Geometry check sheet. Reference: the model listing, model coordinates, mm. Face numbers are marked on the shaded views. A direction names the side the tool comes from. Round coordinates to 2 decimals unless told otherwise and drop trailing zeros. Loops run counter-clockwise (first coordinate to the right, second up) from the corner with the lowest first, then second, coordinate; pieces in that order, holes last. Notation, with made-up numbers: (-2.75, 50.25) -> (18.25, 50.25) arc R20 cw to (18.25, 86.25) -> close; hole circle Ø2 at (30, 10.25). An arc over 180 degrees is marked (long way). Use one line per item in the form item = value.
from build123d import *

# Parameters (mm, degrees)
BOSS_EXTRUDE1_DEPTH = 50
SKETCH2_W           = 25
SKETCH2_H           = 10
CUT_EXTRUDE1_DEPTH  = 84.815273071


with BuildPart() as part:
    # Sketch1 → Boss-Extrude1 (new body)
    with BuildSketch(Plane(origin=(0, 0, 0), x_dir=(0, 0, -1), z_dir=(1, 0, 0))):
        Polygon((0, 0), (30, 0), (30, 10), (20, 10), (20, 20), (50, 20), (50, 10), (40, 10), (40, 0), (70, 0), (70, 30), (45, 30), (45, 50), (25, 50), (25, 30), (0, 30), align=None)
    extrude(amount=-BOSS_EXTRUDE1_DEPTH)

    # Sketch2 → Cut-Extrude1 (cut, through all)
    with BuildSketch(Plane.XY.offset(-25)):
        with Locations((-25, 45)):
            Rectangle(SKETCH2_W, SKETCH2_H)
    extrude(amount=-CUT_EXTRUDE1_DEPTH, mode=Mode.SUBTRACT)


solid = part.part
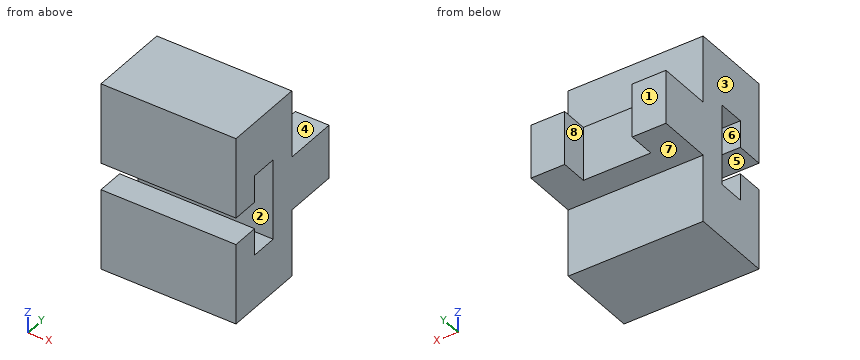
1. Material ranges on line 1 along Z through (x, y) = (-10.5, 17); line 2 along X through (y, z) = (45.5, -39.5); line 3 along Z through (x, y) = (-5, 8.5), recorded low to high.
Return value:
line_1 = -70 to -50, -20 to 0
line_2 = -50 to -37.5, -12.5 to 0
line_3 = -70 to -40, -30 to 0
2. Section check A-A (y = 17.5). Record the boundary of the cut face in (x, z), then the cut area to 3 significant figures.
Return value:
outline = (-50, -70) -> (0, -70) -> (0, -50) -> (-50, -50) -> close; (-50, -20) -> (0, -20) -> (0, 0) -> (-50, 0) -> close
area = 2,000 mm2
3. Section check B-B (z = -21). Record the boundary of the cut face in (x, y), then the cut area to 3 significant figures.
Return value:
outline = (-50, 0) -> (0, 0) -> (0, 10) -> (-50, 10) -> close; (-50, 20) -> (0, 20) -> (0, 30) -> (-50, 30) -> close
area = 1,000 mm2
4. Mould release check, pull along Y, two halves, no side actions. Record for the marked faces 1, 2 and 3: released by +Y, released by -Y, zero draft, split by the parting line, or undercut.
Return value:
face_1 = released by +Y
face_2 = undercut
face_3 = zero draft
5. Section check C-C (x = -30). Record the boundary of the cut face in (y, z), then the cut area to 3 significant figures.
Return value:
outline = (0, -70) -> (30, -70) -> (30, -45) -> (40, -45) -> (40, -25) -> (30, -25) -> (30, 0) -> (0, 0) -> (0, -30) -> (10, -30) -> (10, -20) -> (20, -20) -> (20, -50) -> (10, -50) -> (10, -40) -> (0, -40) -> close
area = 1,900 mm2
6. Tool access check on the marked faces 4, 5, 6, 7 and 8. Record the directions out of +Z, -Z, +X, -X, +Y, -Y that give a thin tool (end or side, any length) a straight path to the whole face; none if there is none.
Return value:
face_4 = +Z, +X, -X, +Y
face_5 = +X, -X, -Y
face_6 = +X, -X
face_7 = -Z, +X, -X, +Y
face_8 = +Z, -Z, +Y
7. Section check D-D (z = -36.5). Record the boundary of the cut face in (x, y).
Return value:
outline = (-50, 20) -> (0, 20) -> (0, 50) -> (-12.5, 50) -> (-12.5, 40) -> (-37.5, 40) -> (-37.5, 50) -> (-50, 50) -> close
8. Gauge pin test, flat ends, axial feed: pin 1 (22 mm diameter, centred on x = -34.5, y = 43.5, fed in from +Z); pin 2 (10 mm diameter, centred on x = -19, z = -31, fed in from +Y); pin 3 (20 mm diameter, centred on x = -28, z = -58.5, fed in from +Y). Record the tip position at first contact, or that the pin passes through.
Return value:
pin_1 = -25
pin_2 = 40
pin_3 = 30
